```python
from build123d import *

# Parameters (mm, degrees)
SKETCH_1_R          = 2.05
SKETCH_1_R_2        = 30
SKETCH_1_W          = 2.8
SKETCH_1_H          = 8.8
EXTRUDE_1_DEPTH     = 2
SKETCH_4_W          = 8
SKETCH_4_H          = 3
SKETCH_4_R          = 1.55
SKETCH_4_R_2        = 2.05
CUT_EXTRUDE_1_DEPTH = 10
FILLET_1_R          = 1.3


with BuildPart() as part:
    # 草图1 → 凸台-拉伸1 (new body)
    with BuildSketch(Plane.XY):
        Polygon((0, 0), (0, -4), (-1.45, -4), (-1.45, -7.2), (0, -7.2), (0, -10.4), (4.1, -10.4), (4.1, -7.2), (5.55, -7.2), (5.55, -4), (4.1, -4), (4.1, 0), (31.05, 0), (31.05, 5), (39.05, 5), (39.05, 0), (66, 0), (66, -4), (64.55, -4), (64.55, -7.2), (66, -7.2), (66, -10.4), (70.1, -10.4), (70.1, -7.2), (71.55, -7.2), (71.55, -4), (70.1, -4), (70.1, 0), (97.05, 0), (97.05, 5), (105.05, 5), (105.05, 0), (132, 0), (144.05, 0), (146.05, 0), (151.05, 0), (151.05, -200), (146.05, -200), (144.05, -200), (132, -200), (105.05, -200), (105.05, -205), (97.05, -205), (97.05, -200), (70.1, -200), (70.1, -196), (71.55, -196), (71.55, -192.8), (70.1, -192.8), (70.1, -189.6), (66, -189.6), (66, -192.8), (64.55, -192.8), (64.55, -196), (66, -196), (66, -200), (39.05, -200), (39.05, -205), (31.05, -205), (31.05, -200), (4.1, -200), (4.1, -196), (5.55, -196), (5.55, -192.8), (4.1, -192.8), (4.1, -189.6), (0, -189.6), (0, -192.8), (-1.45, -192.8), (-1.45, -196), (0, -196), (0, -200), (-26.95, -200), (-26.95, -205), (-34.95, -205), (-34.95, -200), (-61.9, -200), (-61.9, -196), (-60.45, -196), (-60.45, -192.8), (-61.9, -192.8), (-61.9, -189.6), (-66, -189.6), (-66, -192.8), (-67.45, -192.8), (-67.45, -196), (-66, -196), (-66, -200), (-92.95, -200), (-92.95, -205), (-100.95, -205), (-100.95, -200), (-127.9, -200), (-139.95, -200), (-141.95, -200), (-146.95, -200), (-146.95, 0), (-141.95, 0), (-139.95, 0), (-127.9, 0), (-100.95, 0), (-100.95, 5), (-92.95, 5), (-92.95, 0), (-66, 0), (-66, -4), (-67.45, -4), (-67.45, -7.2), (-66, -7.2), (-66, -10.4), (-61.9, -10.4), (-61.9, -7.2), (-60.45, -7.2), (-60.45, -4), (-61.9, -4), (-61.9, 0), (-34.95, 0), (-34.95, 5), (-26.95, 5), (-26.95, 0), align=None)
        with Locations((-141.95, -100)):
            Circle(SKETCH_1_R, mode=Mode.SUBTRACT)
        with Locations(Location((146.05, -100, 0), (0, 0, 180))):
            Circle(SKETCH_1_R, mode=Mode.SUBTRACT)
        with Locations((1.5, -100)):
            Circle(SKETCH_1_R_2, mode=Mode.SUBTRACT)
        with Locations((-141.95, -67)):
            Rectangle(SKETCH_1_W, SKETCH_1_H, mode=Mode.SUBTRACT)
        with Locations((-141.95, -133)):
            Rectangle(SKETCH_1_W, SKETCH_1_H, mode=Mode.SUBTRACT)
        with Locations((146.05, -133)):
            Rectangle(SKETCH_1_W, SKETCH_1_H, mode=Mode.SUBTRACT)
        with Locations((146.05, -67)):
            Rectangle(SKETCH_1_W, SKETCH_1_H, mode=Mode.SUBTRACT)
    extrude(amount=EXTRUDE_1_DEPTH)

    # 草图4 → 切除-拉伸1 (cut)
    with BuildSketch(Plane.XY.offset(2)):
        with BuildLine():
            Line((116.459883662, -15.5), (84.45, -15.5))
            ThreePointArc((84.45, -15.5), (82.45, -17.5), (84.45, -19.5))
            Line((84.45, -19.5), (116.459883662, -19.5))
            ThreePointArc((116.459883662, -19.5), (118.459883662, -17.5), (116.459883662, -15.5))
        make_face()
        with BuildLine():
            ThreePointArc((84.45, -53.5), (82.45, -55.5), (84.45, -57.5))
            Line((84.45, -57.5), (116.459883662, -57.5))
            ThreePointArc((116.459883662, -57.5), (118.459883662, -55.5), (116.459883662, -53.5))
            Line((116.459883662, -53.5), (84.45, -53.5))
        make_face()
        with Locations((-96.95, 3.5)):
            Rectangle(SKETCH_4_W, SKETCH_4_H)
        with Locations((-96.95, -203.5)):
            Rectangle(SKETCH_4_W, SKETCH_4_H)
        with Locations((101.05, 3.5)):
            Rectangle(SKETCH_4_W, SKETCH_4_H)
        with Locations((101.05, -203.5)):
            Rectangle(SKETCH_4_W, SKETCH_4_H)
        with Locations((-75.364854909, -176.46991287)):
            Circle(SKETCH_4_R)
        with Locations((-103.264854909, -176.46991287)):
            Circle(SKETCH_4_R)
        with Locations((-70.264854909, -124.36991287)):
            Circle(SKETCH_4_R)
        with Locations((-115.764854909, -124.36991287)):
            Circle(SKETCH_4_R)
        with Locations((-117.464854909, -35.441983185)):
            Circle(SKETCH_4_R)
        with Locations((-68.464854909, -35.441983185)):
            Circle(SKETCH_4_R)
        with Locations((-117.464854909, -93.441983185)):
            Circle(SKETCH_4_R)
        with Locations((-68.464854909, -93.441983185)):
            Circle(SKETCH_4_R)
        with Locations((-125.55, -17.5)):
            Circle(SKETCH_4_R_2)
        with Locations((-125.55, -55.5)):
            Circle(SKETCH_4_R_2)
        with Locations((-115.55, -55.5)):
            Circle(SKETCH_4_R_2)
        with Locations(Location((-115.55, -17.5, 0), (0, 0, 180))):
            Circle(SKETCH_4_R_2)
        with Locations((-46.95, -150)):
            Circle(SKETCH_4_R_2)
        with Locations((23.05, -150)):
            Circle(SKETCH_4_R_2)
    extrude(amount=-CUT_EXTRUDE_1_DEPTH, mode=Mode.SUBTRACT)

    # 圆角1
    fillet_1_edges = [part.edges().sort_by_distance(p)[0] for p in [
        (31.05, 5, 1),
        (39.05, 5, 1),
        (39.05, -205, 1),
        (31.05, -205, 1),
        (-26.95, -205, 1),
        (-34.95, -205, 1),
        (-34.95, 5, 1),
        (-26.95, 5, 1),
    ]]
    fillet(fillet_1_edges, radius=FILLET_1_R)


solid = part.part
```
Verification items for the finished model (mm, model axes). Coordinates: 2 decimals unless noted, no trailing zeros. Loops run counter-clockwise (first coordinate to the right, second up) from the corner with the lowest first, then second, coordinate; pieces in that order, holes last. Notation, with made-up numbers: (5, 31) -> (22, 31) arc R25 cw to (22, 66) -> close; hole circle Ø2 at (55.25, -25.75). An arc over 180 degrees is marked (long way). Answer in a Markdown table with one row per item.
1) Draft check along Y on faces 1 (the face through (37, -99, 2)), 2 (the face through (-2.405, -70.255, 0.986)). Enter one of: released by +Y, released by -Y, zero draft, split by the parting line, or undercut.
The answers:
| item | result |
|---|---|
| face 1 | zero draft |
| face 2 | undercut |
2) Section check A-A (y = -114). Record the cut outline in (x, z).
The answers:
| item | result |
|---|---|
| outline | (-146.95, 0) -> (-25.03, 0) -> (-25.03, 2) -> (-146.95, 2) -> close; (28.03, 0) -> (151.05, 0) -> (151.05, 2) -> (28.03, 2) -> close |
3) Section check B-B (x = -56). Record the cut outline in (y, z).
The answers:
| item | result |
|---|---|
| outline | (-200, 0) -> (0, 0) -> (0, 2) -> (-200, 2) -> close |
4) Depth check by flat-ended pin: P1, Ø0.6, axis at x = -127.5, z = 1.5, coming from the -Y side; P2, Ø1, axis at x = 146.5, z = 0.5, coming from the +Y side; P3, Ø0.6, axis at x = -95.5, z = 0.5, coming from the +Y side. Enter the tip coordinate at first touch or a pass-through.
The answers:
| item | result |
|---|---|
| P1 | stops at y = -200 |
| P2 | stops at y = 0 |
| P3 | stops at y = 2 |
5) Scan lines: line 1 along Y through (x, z) = (99, 1.8); line 2 along X through (y, z) = (-133.5, 1.6); line 3 along X through (y, z) = (-150, 0.45). Record each from-to range of solid material in increasing order. Write a range as from..to.
The answers:
| item | result |
|---|---|
| line 1 | y = -202..-57.5, -53.5..-19.5, -15.5..2 |
| line 2 | x = -146.95..-143.35, -140.55..144.65, 147.45..151.05 |
| line 3 | x = -146.95..-49, -44.9..21, 25.1..151.05 |
6) Section check C-C (z = 0.95). Give the number of separate pieces and of enclosed holes in the cut face, and give its area (3 significant figures).
The answers:
| item | result |
|---|---|
| separate pieces | 1 |
| enclosed holes | 23 |
| area | 56,100 mm2 |
